Read the model definition and answer for the solid it produces. Units are mm, in the model's axes. Round coordinates to 2 decimals unless told otherwise and drop trailing zeros. Order: outer loops, then holes, each group sorted by start corner. A loop starts at its lowest first (then second) coordinate and runs counter-clockwise, first axis right, second up. Notation, with made-up numbers: (5, 82.25) - (40, 82.25) arc R18 cw to (40, 98.25) - close; hole circle Ø2 at (40, 47.25). An arc over 180 degrees is marked (long way). Answer as a JSON object with one key per item and string values. Group by question number.
Q1. Given pin 1 Ø3 at (x, z) = (-140, -21) entering from -Y; pin 2 Ø2 at (y, z) = (3, 87.5) entering from +X; pin 3 Ø2.5 at (y, z) = (2.5, -104.5) entering from -X, each flat-ended and moving along its own axis, determine where each tip first touches the part or whether it passes through.
Q2. Consider line 1 (X direction, y = 0.2, z = -112); line 2 (Z direction, x = -174.5, y = 3.45); line 3 (Z direction, x = -185, y = 1.45). Determine where each line is inside the solid, lowest interval first.
Q3. A cutting plane is placed at A-A on z = -112.5. Determine the outline of the cut face in (x, y), and give its area (3 significant figures).
Q4. A cutting plane is placed at B-B on y = 1.5. Count the separate pieces of the cut face and the enclosed holes in it, and give its area (3 significant figures).
```python
from build123d import *

# Parameters (mm, degrees)
SKETCH_1_W          = 400
SKETCH_1_H          = 380
EXTRUDE_1_DEPTH     = 5
SKETCH_2_R          = 2.25
SKETCH_2_R_2        = 2.5
SKETCH_2_R_3        = 3
SKETCH_2_R_4        = 2
SKETCH_2_R_5        = 1.5
SKETCH_2_W          = 30
SKETCH_2_H          = 70
SKETCH_2_W_2        = 34
SKETCH_2_H_2        = 50
CUT_EXTRUDE_1_DEPTH = 276.907593226


with BuildPart() as part:
    # 草圖1 → 填料-伸長1 (new body)
    with BuildSketch(Plane(origin=(0, 0, 0), x_dir=(1, 0, 0), z_dir=(0, 1, 0))):
        Rectangle(SKETCH_1_W, SKETCH_1_H)
    extrude(amount=EXTRUDE_1_DEPTH)

    # 草圖2 → 除料-伸長1 (cut, through all)
    with BuildSketch(Plane(origin=(0, 5, 0), x_dir=(1, 0, 0), z_dir=(0, 1, 0))):
        with Locations(Location((-127.07, -24.13, 0), (0, 0, 270))):
            Circle(SKETCH_2_R)
        with Locations(Location((-125.8, 24.13, 0), (0, 0, 270))):
            Circle(SKETCH_2_R)
        with Locations(Location((-74.5, 8.89, 0), (0, 0, 270))):
            Circle(SKETCH_2_R_2)
        with Locations(Location((-185, 145, 0), (0, 0, 270))):
            Circle(SKETCH_2_R_3)
        with Locations(Location((185, 145, 0), (0, 0, 270))):
            Circle(SKETCH_2_R_3)
        with Locations(Location((-185, -145, 0), (0, 0, 90))):
            Circle(SKETCH_2_R_3)
        with Locations(Location((185, -145, 0), (0, 0, 90))):
            Circle(SKETCH_2_R_3)
        with Locations(Location((81.65, 18.35, 0), (0, 0, 270))):
            Circle(SKETCH_2_R_3)
        with Locations(Location((118.35, 18.35, 0), (0, 0, 270))):
            Circle(SKETCH_2_R_3)
        with Locations(Location((81.65, -18.35, 0), (0, 0, 270))):
            Circle(SKETCH_2_R_3)
        with Locations(Location((118.35, -18.35, 0), (0, 0, 270))):
            Circle(SKETCH_2_R_3)
        with Locations(Location((-145, -85, 0), (0, 0, 270))):
            Circle(SKETCH_2_R_4)
        with Locations(Location((-105, -85, 0), (0, 0, 270))):
            Circle(SKETCH_2_R_4)
        with Locations(Location((-145, -125, 0), (0, 0, 270))):
            Circle(SKETCH_2_R_4)
        with Locations(Location((-105, -125, 0), (0, 0, 270))):
            Circle(SKETCH_2_R_4)
        with Locations(Location((105, -85, 0), (0, 0, 270))):
            Circle(SKETCH_2_R_4)
        with Locations(Location((145, -85, 0), (0, 0, 270))):
            Circle(SKETCH_2_R_4)
        with Locations(Location((105, -125, 0), (0, 0, 270))):
            Circle(SKETCH_2_R_4)
        with Locations(Location((145, -125, 0), (0, 0, 270))):
            Circle(SKETCH_2_R_4)
        with Locations(Location((-145, 125, 0), (0, 0, 270))):
            Circle(SKETCH_2_R_4)
        with Locations(Location((-105, 125, 0), (0, 0, 270))):
            Circle(SKETCH_2_R_4)
        with Locations(Location((-145, 85, 0), (0, 0, 270))):
            Circle(SKETCH_2_R_4)
        with Locations(Location((-105, 85, 0), (0, 0, 270))):
            Circle(SKETCH_2_R_4)
        with Locations(Location((105, 125, 0), (0, 0, 270))):
            Circle(SKETCH_2_R_4)
        with Locations(Location((145, 125, 0), (0, 0, 270))):
            Circle(SKETCH_2_R_4)
        with Locations(Location((105, 85, 0), (0, 0, 270))):
            Circle(SKETCH_2_R_4)
        with Locations(Location((145, 85, 0), (0, 0, 270))):
            Circle(SKETCH_2_R_4)
        with Locations(Location((-42.5, -1.5, 0), (0, 0, 270))):
            Circle(SKETCH_2_R_5)
        with Locations(Location((42.5, -1.5, 0), (0, 0, 270))):
            Circle(SKETCH_2_R_5)
        with Locations(Location((-42.5, -108.5, 0), (0, 0, 270))):
            Circle(SKETCH_2_R_5)
        with Locations(Location((42.5, -108.5, 0), (0, 0, 270))):
            Circle(SKETCH_2_R_5)
        with Locations((185, -95)):
            Rectangle(SKETCH_2_W, SKETCH_2_H)
        with Locations((-185, 95)):
            Rectangle(SKETCH_2_W, SKETCH_2_H)
        with Locations((-185, -95)):
            Rectangle(SKETCH_2_W, SKETCH_2_H)
        with Locations((185, 95)):
            Rectangle(SKETCH_2_W, SKETCH_2_H)
        with Locations((-125, -105)):
            Rectangle(SKETCH_2_W_2, SKETCH_2_H_2)
        with Locations((125, -105)):
            Rectangle(SKETCH_2_W_2, SKETCH_2_H_2)
        with Locations((-125, 105)):
            Rectangle(SKETCH_2_W_2, SKETCH_2_H_2)
        with Locations((125, 105)):
            Rectangle(SKETCH_2_W_2, SKETCH_2_H_2)
        Polygon((-21.15, 85.5), (-15.5, 91.15), (15.5, 91.15), (21.15, 85.5), (21.15, 54.5), (15.5, 48.85), (-15.5, 48.85), (-21.15, 54.5), align=None)
        with BuildLine():
            Line((-214.88693476, -145), (-214.88693476, -175))
            ThreePointArc((-214.88693476, -175), (-234.88693476, -195), (-254.88693476, -175))
            Line((-254.88693476, -175), (-254.88693476, -145))
            ThreePointArc((-254.88693476, -145), (-234.88693476, -125), (-214.88693476, -145))
        make_face()
        with BuildLine():
            Line((-214.88693476, 145), (-214.88693476, 175))
            ThreePointArc((-214.88693476, 175), (-234.88693476, 195), (-254.88693476, 175))
            Line((-254.88693476, 175), (-254.88693476, 145))
            ThreePointArc((-254.88693476, 145), (-234.88693476, 125), (-214.88693476, 145))
        make_face()
        with BuildLine():
            Line((214.88693476, -145), (214.88693476, -175))
            ThreePointArc((214.88693476, -175), (234.88693476, -195), (254.88693476, -175))
            Line((254.88693476, -175), (254.88693476, -145))
            ThreePointArc((254.88693476, -145), (234.88693476, -125), (214.88693476, -145))
        make_face()
        with BuildLine():
            Line((214.88693476, 145), (214.88693476, 175))
            ThreePointArc((214.88693476, 175), (234.88693476, 195), (254.88693476, 175))
            Line((254.88693476, 175), (254.88693476, 145))
            ThreePointArc((254.88693476, 145), (234.88693476, 125), (214.88693476, 145))
        make_face()
        with BuildLine():
            Line((-147.5, 181), (-102.5, 181))
            ThreePointArc((-102.5, 181), (-96.5, 175), (-102.5, 169))
            Line((-102.5, 169), (-147.5, 169))
            ThreePointArc((-147.5, 169), (-153.5, 175), (-147.5, 181))
        make_face()
        with BuildLine():
            Line((-147.5, -181), (-102.5, -181))
            ThreePointArc((-102.5, -181), (-96.5, -175), (-102.5, -169))
            Line((-102.5, -169), (-147.5, -169))
            ThreePointArc((-147.5, -169), (-153.5, -175), (-147.5, -181))
        make_face()
        with BuildLine():
            Line((147.5, 181), (102.5, 181))
            ThreePointArc((102.5, 181), (96.5, 175), (102.5, 169))
            Line((102.5, 169), (147.5, 169))
            ThreePointArc((147.5, 169), (153.5, 175), (147.5, 181))
        make_face()
        with BuildLine():
            Line((147.5, -181), (102.5, -181))
            ThreePointArc((102.5, -181), (96.5, -175), (102.5, -169))
            Line((102.5, -169), (147.5, -169))
            ThreePointArc((147.5, -169), (153.5, -175), (147.5, -181))
        make_face()
    extrude(amount=-CUT_EXTRUDE_1_DEPTH, mode=Mode.SUBTRACT)


solid = part.part
```
Result set:
{
 "1": {"pin 1": "stops at y = 0", "pin 2": "stops at x = 170", "pin 3": "stops at x = -170"},
 "2": {"line 1": "x = -170 to -142, -108 to 108, 142 to 170", "line 2": "z = -190 to -130, -60 to 60, 130 to 190", "line 3": "z = -190 to -148, -142 to -130, -60 to 60, 130 to 142, 148 to 190"},
 "3": {"outline": "(-170, 0) - (-142, 0) - (-142, 5) - (-170, 5) - close; (-108, 0) - (108, 0) - (108, 5) - (-108, 5) - close; (142, 0) - (170, 0) - (170, 5) - (142, 5) - close", "area": "1,360 mm²"},
 "4": {"separate pieces": "1", "enclosed holes": "40", "area": "132,000 mm²"}
}
